Input: part model. Units: mm. Frame: model coordinates. A direction names the side the tool comes from. Round coordinates to 2 decimals unless told otherwise and drop trailing zeros. Loops run counter-clockwise (first coordinate to the right, second up) from the corner with the lowest first, then second, coordinate; pieces in that order, holes last. Notation, with made-up numbers: M 41,8.5 L 80,8.5 A24 ccw 80,37.5 Z; hole C 48,45 d6. An arc over 180 degrees is marked long. Use one line per item in the form item = value. Start each with the question number.
Q1. First-contact query: P1, Ø10, axis at x = -29.5, z = 48, coming from the +Y side; P2, Ø4, axis at x = -17, z = 20, coming from the -Y side; P3, Ø8, axis at y = -13.5, z = 39, coming from the -X side; P4, Ø6, axis at y = 0, z = 37, coming from the +X side. Flat tips, straight axial feed; report the tip coordinate or a pass-through.
Q2. Section query B-B, the plane y = 0. Output: boundary loops of the cut face in (x, z).
Q3. Section query D-D, the plane z = 16.5. Output: boundary loops of the cut face in (x, y).
Q4. Ray query, line 1 along X through (y, z) = (10, 33); line 2 along Y through (x, z) = (-36.2, 3.5); line 3 along Z through (x, y) = (-19, 19). Return the intervals inside material, ascending.
Q5. Access query for faces 4 (the flat face through (-10, 26, 10)), 5 (the flat face through (-0.4, 20.7, 14.7)), 6 (the flat face through (-28.7, 0, 34)), 7 (the flat face through (28.7, 0, 34)), 8 (the flat face through (0, 0, 15)). Directions: +Z, -Z, +X, -X, +Y, -Y. A direction counts if a zero-diameter tool reaches every point of the face in a straight line with its end or side. Return the directions, or none.
Q6. Section query A-A, the plane z = 9. Output: boundary loops of the cut face in (x, y), and give its area (3 significant figures).
Q7. Mould query, pull axis X, two halves, no side actions, for faces 1 (the cylindrical face through (24.756, 0.455, 57.695)), 2 (the cylindrical face through (-33.815, -9.949, 5.07)), 3 (the cylindrical face through (-40.85, -17.69, 5.07)). Classes: pulls with the +X half, pulls with the -X half, needs draft (parallel to the pull), parting line crosses it, or undercut.
Q8. Section query C-C, the plane x = -27. Output: boundary loops of the cut face in (y, z).
```python
from build123d import *

# Parameters (mm, degrees)
SKETCH1_W           = 57.4
SKETCH1_H           = 41.4
BOSS_EXTRUDE1_DEPTH = 10
SKETCH2_W           = 57.4
SKETCH2_H           = 41.4
BOSS_EXTRUDE2_DEPTH = 5
BOSS_EXTRUDE3_DEPTH = 8
BOSS_EXTRUDE4_START = -8
BOSS_EXTRUDE4_DEPTH = 8
CUT_EXTRUDE1_REACH  = 85.979
SKETCH6_R           = 2.5
SKETCH11_W          = 10
SKETCH11_H          = 41.4
BOSS_EXTRUDE5_DEPTH = 15
SKETCH12_W          = 10
SKETCH12_H          = 41.4
BOSS_EXTRUDE6_DEPTH = 15
SKETCH13_W          = 87.4
SKETCH13_H          = 10
BOSS_EXTRUDE7_DEPTH = 15
SKETCH14_R          = 2.5
CUT_EXTRUDE2_DEPTH  = 10
FILLET1_R           = 10


with BuildPart() as part:
    # Sketch1 → Boss-Extrude1 (new body)
    with BuildSketch(Plane.XY):
        Rectangle(SKETCH1_W, SKETCH1_H)
    extrude(amount=BOSS_EXTRUDE1_DEPTH)

    # Sketch2 → Boss-Extrude2 (add)
    with BuildSketch(Plane.XY.offset(10)):
        Rectangle(SKETCH2_W, SKETCH2_H)
    extrude(amount=BOSS_EXTRUDE2_DEPTH)

    # Sketch4 → Boss-Extrude3 (add)
    with BuildSketch(Plane(origin=(28.7, 0, 0), x_dir=(0, 0, -1), z_dir=(1, 0, 0))):
        with BuildLine():
            Line((-15, -20.7), (-15, 20.7))
            Line((-15, 20.7), (-37, 20.7))
            ThreePointArc((-37, 20.7), (-57.7, 0), (-37, -20.7))
            Line((-37, -20.7), (-15, -20.7))
        make_face()
    extrude(amount=-BOSS_EXTRUDE3_DEPTH)

    # Sketch5 → Boss-Extrude4 (add)
    with BuildSketch(Plane.ZY.offset(28.7).offset(BOSS_EXTRUDE4_START)):
        with BuildLine():
            Line((15, 20.7), (15, -20.7))
            Line((15, -20.7), (37, -20.7))
            ThreePointArc((37, -20.7), (57.7, 0), (37, 20.7))
            Line((37, 20.7), (15, 20.7))
        make_face()
    extrude(amount=BOSS_EXTRUDE4_DEPTH)

    # Cut-Extrude1: up to this face of the body (flat: up to its plane)
    cut_extrude1_end = Plane(part.part.faces().sort_by_distance((-28.7, 0, 26.829272143))[0])
    # Sketch6 → Cut-Extrude1 (cut, up to the picked face)
    with BuildSketch(Plane(origin=(28.7, 0, 0), x_dir=(0, 0, -1), z_dir=(1, 0, 0)), mode=Mode.PRIVATE) as cut_extrude1_sk1:
        with Locations((-37, 0)):
            Circle(SKETCH6_R)
    cut_extrude1_tool1 = split(extrude(cut_extrude1_sk1.sketch, amount=-CUT_EXTRUDE1_REACH, mode=Mode.PRIVATE), bisect_by=cut_extrude1_end, keep=Keep.BOTH, mode=Mode.PRIVATE)
    add(cut_extrude1_tool1.solids().sort_by(Axis((28.7, 0, 37), (-1, 0, 0)))[0], mode=Mode.SUBTRACT)

    # Sketch11 → Boss-Extrude5 (add)
    with BuildSketch(Plane.ZY.offset(28.7)):
        with Locations((5, 0)):
            Rectangle(SKETCH11_W, SKETCH11_H)
    extrude(amount=BOSS_EXTRUDE5_DEPTH)

    # Sketch12 → Boss-Extrude6 (add)
    with BuildSketch(Plane(origin=(28.7, 0, 0), x_dir=(0, 0, -1), z_dir=(1, 0, 0))):
        with Locations((-5, 0)):
            Rectangle(SKETCH12_W, SKETCH12_H)
    extrude(amount=BOSS_EXTRUDE6_DEPTH)

    # Sketch13 → Boss-Extrude7 (add)
    with BuildSketch(Plane(origin=(0, 20.7, 0), x_dir=(1, 0, 0), z_dir=(0, 1, 0))):
        with Locations((0, -5)):
            Rectangle(SKETCH13_W, SKETCH13_H)
    extrude(amount=BOSS_EXTRUDE7_DEPTH)

    # Sketch14 → Cut-Extrude2 (cut)
    with BuildSketch(Plane.XY.offset(10)):
        with Locations((-36.2, -10.7)):
            Circle(SKETCH14_R)
        with Locations((-36.2, 28.2)):
            Circle(SKETCH14_R)
        with Locations((36.2, 28.2)):
            Circle(SKETCH14_R)
        with Locations((36.2, -10.7)):
            Circle(SKETCH14_R)
        with Locations((0, 28.2)):
            Circle(SKETCH14_R)
    extrude(amount=-CUT_EXTRUDE2_DEPTH, mode=Mode.SUBTRACT)

    # Fillet1
    fillet1_edges = [part.edges().sort_by_distance(p)[0] for p in [
        (-43.7, -20.7, 5),
        (43.7, -20.7, 5),
        (-43.7, 35.7, 5),
        (43.7, 35.7, 5),
    ]]
    fillet(fillet1_edges, radius=FILLET1_R)


solid = part.part
```
Results found:
q1.P1 = 19.79
q1.P2 = through
q1.P3 = -28.7
q1.P4 = 28.7
q2.outline = M -43.7,0 L 43.7,0 L 43.7,10 L 28.7,10 L 28.7,34.5 L 20.7,34.5 L 20.7,15 L -20.7,15 L -20.7,34.5 L -28.7,34.5 L -28.7,10 L -43.7,10 Z; M -28.7,39.5 L -20.7,39.5 L -20.7,57.7 L -28.7,57.7 Z; M 20.7,39.5 L 28.7,39.5 L 28.7,57.7 L 20.7,57.7 Z
q3.outline = M -28.7,-20.7 L -20.7,-20.7 L -20.7,20.7 L -28.7,20.7 Z; M 20.7,-20.7 L 28.7,-20.7 L 28.7,20.7 L 20.7,20.7 Z
q4.line_1 = -28.7 to -20.7, 20.7 to 28.7
q4.line_2 = -20.38 to -13.2, -8.2 to 25.7, 30.7 to 35.38
q4.line_3 = 0 to 15
q5.face_4 = +Z, +Y
q5.face_5 = +Z, +X, -X, +Y
q5.face_6 = +Z, -X, +Y, -Y
q5.face_7 = +Z, +X, +Y, -Y
q5.face_8 = +Z, +Y, -Y
q6.outline = M -43.7,-10.7 A10 ccw -33.7,-20.7 L 33.7,-20.7 A10 ccw 43.7,-10.7 L 43.7,25.7 A10 ccw 33.7,35.7 L -33.7,35.7 A10 ccw -43.7,25.7 Z; hole C -36.2,-10.7 d5; hole C -36.2,28.2 d5; hole C 0,28.2 d5; hole C 36.2,-10.7 d5; hole C 36.2,28.2 d5
q6.area = 4,750 mm²
q7.face_1 = needs draft
q7.face_2 = undercut
q7.face_3 = pulls with the -X half
q8.outline = M -20.7,0 L 35.7,0 L 35.7,10 L 20.7,10 L 20.7,37 A20.7 ccw -20.7,37 Z; hole C 0,37 d5
